from build123d import *

# Parameters (mm, degrees)
F0_R      = 40
F0_R_2    = 35
F1_DEPTH  = 700
F3_R      = 44
F3_R_2    = 39.15
F4_DEPTH  = 2.5
F6_R      = 42.5
F6_R_2    = 39.15
F7_DEPTH  = 2.5
F10_R     = 42.5
F10_R_2   = 39.15
F11_DEPTH = 2.5
F13_R     = 42.5
F13_R_2   = 39.15
F14_DEPTH = 2.5
F16_R     = 44
F16_R_2   = 39.15
F17_DEPTH = 2.5
F19_R     = 44
F19_R_2   = 39.15
F20_DEPTH = 2.5


with BuildPart() as f1:
    # F0 (on Front) → F1 (new body)
    with BuildSketch(Plane.XZ):
        Circle(F0_R)
        Circle(F0_R_2, mode=Mode.SUBTRACT)
    extrude(amount=F1_DEPTH)

    # F3 (on offset) → F4 (cut)
    with BuildSketch(Plane.XZ.offset(20)):
        Circle(F3_R)
        Circle(F3_R_2, mode=Mode.SUBTRACT)
    extrude(amount=F4_DEPTH, mode=Mode.SUBTRACT)

    # F6 (on offset) → F7 (cut)
    with BuildSketch(Plane.XZ.offset(55.5)):
        Circle(F6_R)
        Circle(F6_R_2, mode=Mode.SUBTRACT)
    extrude(amount=F7_DEPTH, mode=Mode.SUBTRACT)

    # F10 (on offset) → F11 (cut)
    with BuildSketch(Plane.XZ.offset(480)):
        Circle(F10_R)
        Circle(F10_R_2, mode=Mode.SUBTRACT)
    extrude(amount=-F11_DEPTH, mode=Mode.SUBTRACT)

    # F13 (on offset) → F14 (cut)
    with BuildSketch(Plane.XZ.offset(444.5)):
        Circle(F13_R)
        Circle(F13_R_2, mode=Mode.SUBTRACT)
    extrude(amount=-F14_DEPTH, mode=Mode.SUBTRACT)

    # F16 (on offset) → F17 (cut)
    with BuildSketch(Plane.XZ.offset(590)):
        Circle(F16_R)
        Circle(F16_R_2, mode=Mode.SUBTRACT)
    extrude(amount=-F17_DEPTH, mode=Mode.SUBTRACT)

    # F19 (on offset) → F20 (cut)
    with BuildSketch(Plane.XZ.offset(600)):
        Circle(F19_R)
        Circle(F19_R_2, mode=Mode.SUBTRACT)
    extrude(amount=-F20_DEPTH, mode=Mode.SUBTRACT)


solid = f1.part
Input: part model. Units: mm. Frame: model coordinates. A direction names the side the tool comes from. Round coordinates to 2 decimals unless told otherwise and drop trailing zeros. Write each loop counter-clockwise with the first axis right and the second up, starting at its lowest first coordinate (ties: lowest second). Pieces come first, ordered by that corner, then holes.
1) Draft query along Z for faces 1 (the flat face through (29.4, -442, -26.5)), 2 (the cylindrical face through (-28, -345, -21)), 3 (the cylindrical face through (36.165, -56.732, -14.995)). Return one class per face: pulls with the +Z half, pulls with the -Z half, needs draft (parallel to the pull), parting line crosses it, or undercut.
2) Cut plane A-A (y = -106). Return the cut outline in (x, z).
3) Reachability of faces 4 (the flat face through (29.4, -480, -26.5)), 5 (the cylindrical face through (-8.67, -533, -39.05)) from +Z, -Z, +X, -X, +Y, -Y: full face, straight path, thin tool, end or side. Return the list, or none.
4) Ray query, L1, parallel to Z at x = 1, y = -620; L2, parallel to Z at x = -6, y = -27.5. Return the intervals inside material, ascending.
5) Contact query for flat-ended pins moving along their axis: P1, Ø10, axis at y = -302, z = 0.5, coming from the +X side; P2, Ø6, axis at x = 1.5, y = -168, coming from the +Z side; P3, Ø12, axis at y = -309.5, z = -13.5, coming from the +X side; P4, Ø24, axis at x = -8, z = -12.5, coming from the -Y side. Output: stop coordinate, or through.
Geometry says:
1. face 1: needs draft
1. face 2: undercut
1. face 3: parting line crosses it
2. outline: circle Ø80 at (0, 0); hole circle Ø70 at (0, 0)
3. face 4: none
3. face 5: +Y, -Y
4. L1: z = -39.99 to -34.99, 34.99 to 39.99
4. L2: z = -39.55 to -34.48, 34.48 to 39.55
5. P1: stops at x = 40
5. P2: stops at z = 40
5. P3: stops at x = 39.29
5. P4: passes through
